Work out the finished part from the listing and answer in its coordinate system (mm). A direction names the side the tool comes from. Round coordinates to 2 decimals unless told otherwise and drop trailing zeros. Order: outer loops, then holes, each group sorted by start corner. A loop starts at its lowest first (then second) coordinate and runs counter-clockwise, first axis right, second up. Notation, with made-up numbers: (56.25, 12.5) -> (72.25, 12.5) arc R19 cw to (72.25, 41.5) -> close; hole circle Ø3 at (-23, -2.75). An arc over 180 degrees is marked (long way). Use a Markdown table: item, result. Add a question column.
Item 1: A cutting plane is placed at B-B, the plane x = 5. Determine the outline of the cut face in (y, z), plus the area to 3 significant figures.
Item 2: A tool of negligible diameter and unlimited length cuts with its end or side. For faces 1 (the flat face through (0, 7.6, 3)), 2 (the flat face through (-6, 0, 6)), 3 (the flat face through (0, -7.6, 3)), from which of +Z, -Z, +X, -X, +Y, -Y can it reach the whole face along a straight path? Write none if from no direction.
Item 3: Find the intervals of material crossed by L1, parallel to Z at x = -4.5, y = 6.25; L2, parallel to Y at x = 3.5, z = 4.75; L3, parallel to X at y = -4.75, z = 7.5, in increasing order. Write a range as [from, to].
Item 4: A cutting plane is placed at A-A, the plane z = 4.25. Determine the outline of the cut face in (x, y).
Item 5: Flat-ended cylindrical pins translate along their axes: P1, Ø3, axis at x = 6.5, y = 0, coming from the +Z side; P2, Ø1.5, axis at y = 4, z = 3.5, coming from the -X side; P3, Ø6, axis at y = 3.5, z = 3, coming from the -X side; P4, Ø6, axis at x = 6.5, y = -4, coming from the -Z side. Find the tip coordinate at first contact, or state that the pin passes through.
from build123d import *

# Parameters (mm, degrees)
F1_DEPTH = 6
F2_W     = 4
F2_H     = 15.2
F3_DEPTH = 10
F3_TAPER = -3
F4_R     = 2
F5_SIZE  = 0.3


with BuildPart() as f1:
    # F0 (on Top) → F1 (new body)
    with BuildSketch(Plane.XY):
        Polygon((4.3878620458, -7.6), (8.7757240917, 0), (4.3878620458, 7.6), (-4.3878620458, 7.6), (-8.7757240917, 0), (-4.3878620458, -7.6), align=None)
    extrude(amount=F1_DEPTH)

    # F2 (on face) → F3 (join)
    with BuildSketch(Plane.XY.offset(6)):
        Rectangle(F2_W, F2_H)
    extrude(amount=F3_DEPTH, taper=F3_TAPER)

    # F4
    f4_edges = [f1.edges().sort_by_distance(p)[0] for p in [
        (2, 0, 6),
        (-2, 0, 6),
    ]]
    fillet(f4_edges, radius=F4_R)

    # F5
    f5_edges = [f1.edges().sort_by_distance(p)[0] for p in [
        (-6.581793, -3.8, 0),
        (0, -7.6, 0),
        (6.581793, -3.8, 0),
        (6.581793, 3.8, 0),
        (0, 7.6, 0),
        (-6.581793, 3.8, 0),
    ]]
    chamfer(f5_edges, length=F5_SIZE)


solid = f1.part
Reported:
| question | item | result |
|---|---|---|
| 1 | outline | (-6.54, 0.3) -> (-5.94, 0) -> (5.94, 0) -> (6.54, 0.3) -> (6.54, 6) -> (-6.54, 6) -> close |
| 1 | area | 78.3 mm² |
| 2 | face 1 | -Z, +X, -X, +Y |
| 2 | face 2 | +Z, -X, +Y, -Y |
| 2 | face 3 | -Z, +X, -X, -Y |
| 3 | L1 | [0, 6] |
| 3 | L2 | [-7.6, 7.6] |
| 3 | L3 | [-2.17, 2.17] |
| 4 | outline | (-8.78, 0) -> (-4.39, -7.6) -> (4.39, -7.6) -> (8.78, 0) -> (4.39, 7.6) -> (-4.39, 7.6) -> close |
| 5 | P1 | z = 6 |
| 5 | P2 | x = -6.9 |
| 5 | P3 | x = -8.49 |
| 5 | P4 | z = 0 |
